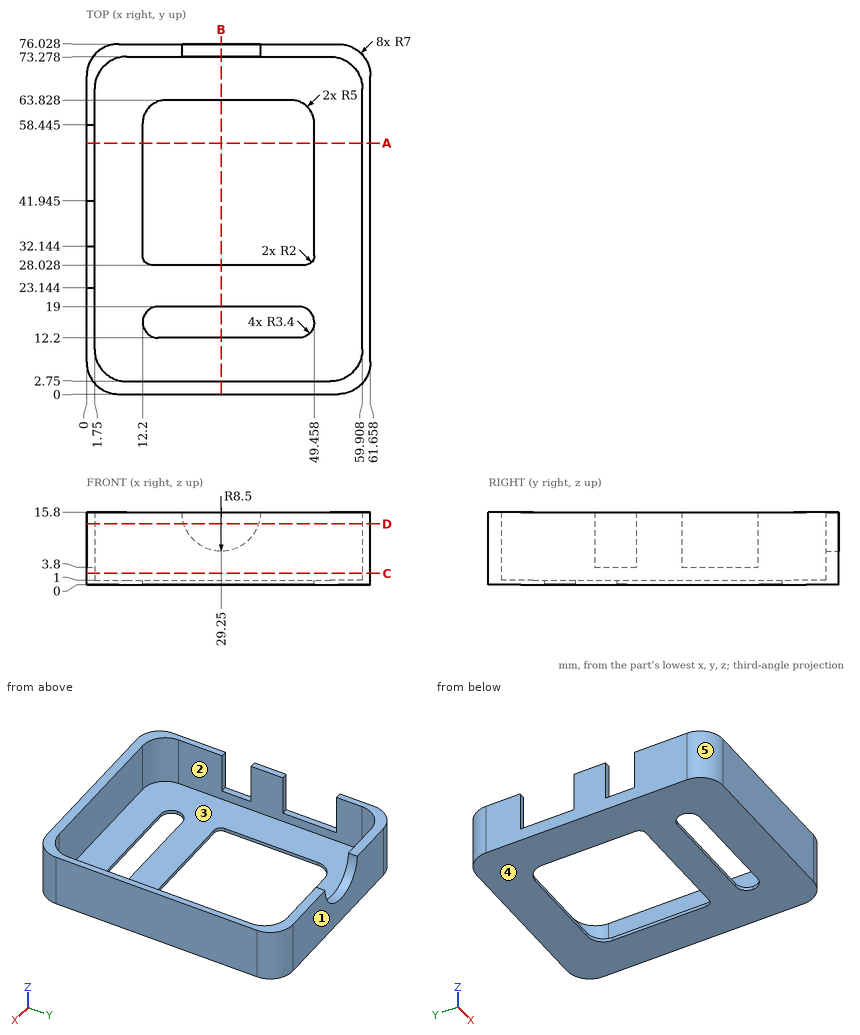
Could you check a few things on this drawing? It's one solid part, dimensions in mm from its lowest x, y, z. A direction names the side the tool comes from. Coordinates: 2 decimals unless noted, no trailing zeros. Write each loop counter-clockwise with the first axis right and the second up, starting at its lowest first coordinate (ties: lowest second). Pieces come first, ordered by that corner, then holes. Notation, with made-up numbers: (6.25, 53) - (11.25, 53) arc R18 ccw to (11.25, 57) - close; hole circle Ø8 at (-16, -27.75). An arc over 180 degrees is marked (long way). Put each result on its own line as item: value. Start each with the question number.
Q1. Thinking about a two-plate mould opening in Y: for the marked faces 3, 4 and 5, which applies, pulls with the +Y half, pulls with the -Y half, needs draft (parallel to the pull), parting line crosses it, or undercut?
Q2. Which directions (+Z, -Z, +X, -X, +Y, -Y) give clear straight access to the entire face, cutting with the end or side of a thin tool? Please do the marked faces 1 and 2.
Q3. Please list where these lines run through material, in increasing order: L1, parallel to Y at x = 13.5, z = 8.5; L2, parallel to X at y = 56, z = 2; L3, parallel to Z at x = 8.5, y = 7.
Q4. I want a section at A-A on y = 54.5. Write out the boundary of the cut face in (x, z).
Q5. I'm going to push flat-ended pins straight in: P1, Ø1.9, axis at x = 1, z = 12, coming from the -Y side; P2, Ø1.4, axis at x = 1, z = 8.5, coming from the +Y side; P3, Ø1.9, axis at x = 0.5, y = 26, coming from the +Z side. Where does each tip first touch, or does it pass through?
Q6. I want a section at B-B on x = 29.25. Write out the boundary of the cut face in (y, z).
Q7. I want a section at C-C on z = 2.5. Write out the boundary of the cut face in (x, y), plus the area to 3 significant figures.
Q8. I want a section at D-D on z = 13.25. Count the separate pieces of the cut face and the enclosed holes in it.
Checks:
1. face 3: undercut
1. face 4: needs draft
1. face 5: pulls with the -Y half
2. face 1: +Z, -Z, +X, -X, +Y
2. face 2: +Z
3. L1: 0 to 2.75, 73.28 to 76.03
3. L2: 0 to 1.75, 59.91 to 61.66
3. L3: 0 to 1
4. outline: (0, 0) - (12.2, 0) - (12.2, 1) - (1.75, 1) - (1.75, 3.8) - (0, 3.8) - close; (49.46, 0) - (61.66, 0) - (61.66, 15.8) - (59.91, 15.8) - (59.91, 1) - (49.46, 1) - close
5. P1: y = 2.15
5. P2: y = 73.6
5. P3: z = 3.8
6. outline: (0, 0) - (12.2, 0) - (12.2, 1) - (2.75, 1) - (2.75, 15.8) - (0, 15.8) - close; (19, 0) - (28.03, 0) - (28.03, 1) - (19, 1) - close; (63.83, 0) - (76.03, 0) - (76.03, 7.3) - (73.28, 7.3) - (73.28, 1) - (63.83, 1) - close
7. outline: (0, 7) arc R7 ccw to (7, 0) - (54.66, 0) arc R7 ccw to (61.66, 7) - (61.66, 69.03) arc R7 ccw to (54.66, 76.03) - (7, 76.03) arc R7 ccw to (0, 69.03) - close; hole (1.75, 9.75) arc R7 ccw to (8.75, 2.75) - (52.91, 2.75) arc R7 ccw to (59.91, 9.75) - (59.91, 66.28) arc R7 ccw to (52.91, 73.28) - (8.75, 73.28) arc R7 ccw to (1.75, 66.28) - close
7. area: 586 mm²
8. separate pieces: 3
8. enclosed holes: 0
